Geometry: see drawing. Coordinates: mm, zero at the bounding-box minimum. A direction names the side the tool comes from. Give positions to 0.01 mm unless a question says otherwise; leave off trailing zeros. Write each loop counter-clockwise with the first axis right and the second up, starting at its lowest first coordinate (ties: lowest second). Pieces come first, ordered by that corner, then holes. Notation, with made-up numbers: (-13, -28.5) -> (22, -28.5) arc R13 cw to (22, -12.5) -> close; hole circle Ø2 at (-39, -0.5). An arc over 180 degrees is marked (long way). Answer as a JSON object with one key per item and string values. Group by question number.
Item 1: Section query A-A on x = 32. Return the cut outline in (y, z), plus the area to 3 significant figures.
Item 2: First-contact query: pin 1 Ø4 at (x, y) = (97, 2) entering from -Z; pin 2 Ø10.5 at (y, z) = (20, 32.5) entering from -X; pin 3 Ø1.5 at (x, y) = (122, 7) entering from +Z; pin 4 Ø25 at (x, z) = (89.5, 60) entering from +Y. Flat tips, straight axial feed; report the tip coordinate or a pass-through.
Item 3: Section query D-D on y = 15. Return the cut outline in (x, z), plus the area to 3 significant figures.
Item 4: Section query C-C on z = 62. Return the cut outline in (x, y).
Item 5: Ray query, probe 1 along X at (y, z) = (1.95, 50); probe 2 along X at (y, z) = (9, 31.5); probe 3 along Y at (x, z) = (29.5, 36). Return the intervals inside material, ascending. Write a range as from..to.
Item 6: Section query B-B on z = 50. Return the cut outline in (x, y).
Item 7: Access query for the marked faces 1 and 2. Directions: +Z, -Z, +X, -X, +Y, -Y. A direction counts if a zero-diameter tool reaches every point of the face in a straight line with its end or side. Return the directions, or none.
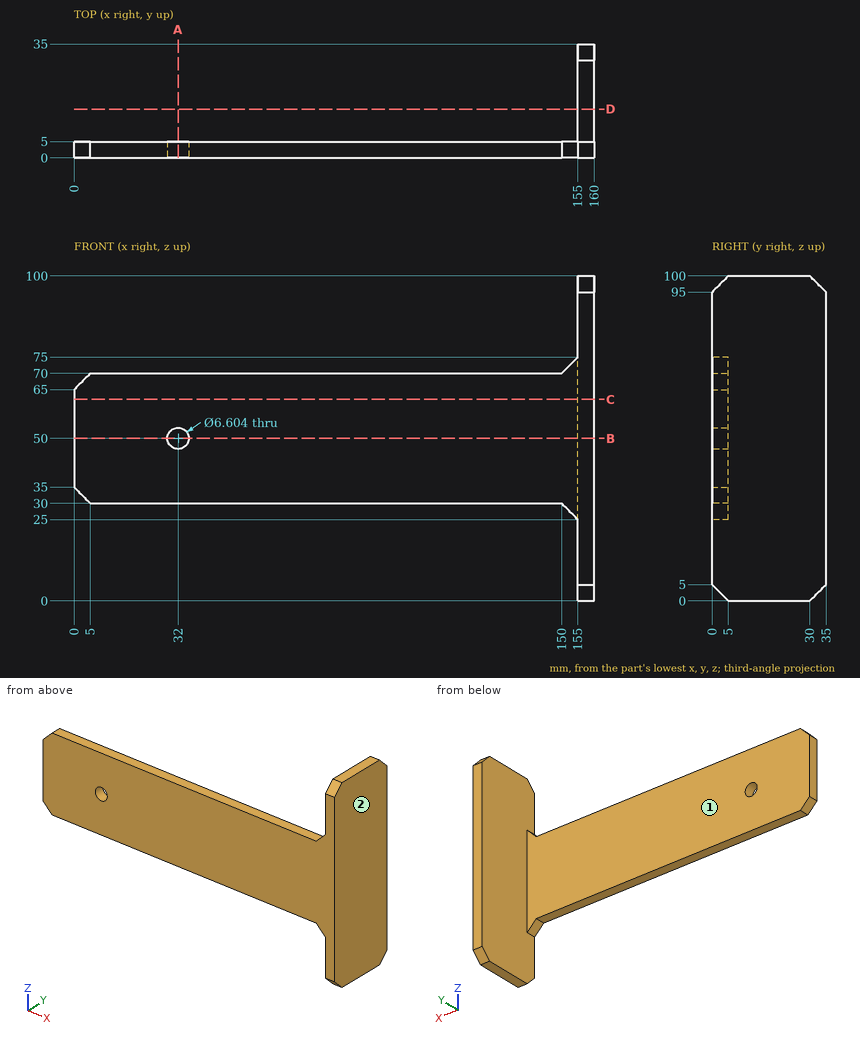
Worked answers:
{
 "1": {"outline": "(0, 30) -> (5, 30) -> (5, 46.7) -> (0, 46.7) -> close; (0, 53.3) -> (5, 53.3) -> (5, 70) -> (0, 70) -> close", "area": "167 mm^2"},
 "2": {"pin 1": "z = 30", "pin 2": "x = 155", "pin 3": "through", "pin 4": "y = 5"},
 "3": {"outline": "(155, 0) -> (160, 0) -> (160, 100) -> (155, 100) -> close", "area": "500 mm^2"},
 "4": {"outline": "(0, 0) -> (160, 0) -> (160, 35) -> (155, 35) -> (155, 5) -> (0, 5) -> close"},
 "5": {"probe 1": "0..28.7, 35.3..160", "probe 2": "155..160", "probe 3": "0..5"},
 "6": {"outline": "(0, 0) -> (28.7, 0) -> (28.7, 5) -> (0, 5) -> close; (35.3, 0) -> (160, 0) -> (160, 35) -> (155, 35) -> (155, 5) -> (35.3, 5) -> close"},
 "7": {"face 1": "+Z, -Z, -X, +Y", "face 2": "+Z, -Z, +X, +Y, -Y"}
}
